from build123d import *

# Parameters (mm, degrees)
F3_DEPTH = 10
F4_R     = 5
F5_SIZE  = 15


# Not quite as in the source:
# - a fillet or chamfer that OpenCascade refuses, or shapes differently, is made with other operations: its cross-section is extruded or revolved along the edge and cut away or added


with BuildPart() as f1:
    # F0 (on Front) → F1 (revolve)
    with BuildSketch(Plane.XZ):
        Polygon((-30, 0), (0, 0), (0, 90), (-20, 90), (-20, 100), (-30, 100), (-30, 75), (-11.7123959959, 75), (-11.7123959959, 20), (-30, 20), align=None)
    revolve(axis=Axis((0, 0, 45), (0, 0, -1)))

    # F2 (on face) → F3 (cut)
    with BuildSketch(Plane.XY.offset(100)):
        with BuildLine():
            ThreePointArc((-3.2492678477, 18.4275136719), (0, 18.7117877734), (3.2492678477, 18.4275136719))
            Line((3.2492678477, 18.4275136719), (5.5579839553, 31.5208933594))
            ThreePointArc((5.5579839553, 31.5208933594), (0, 32.0071539476), (-5.5579839553, 31.5208933594))
            Line((-5.5579839553, 31.5208933594), (-3.2492678477, 18.4275136719))
        make_face()
        with BuildLine():
            ThreePointArc((-15.3277992068, 10.7326405488), (-13.2312320227, 13.2312320227), (-10.7326405488, 15.3277992068))
            Line((-10.7326405488, 15.3277992068), (-18.358549299, 26.218725588))
            ThreePointArc((-18.358549299, 26.218725588), (-22.6324756028, 22.6324756028), (-26.218725588, 18.358549299))
            Line((-26.218725588, 18.358549299), (-15.3277992068, 10.7326405488))
        make_face()
        with BuildLine():
            ThreePointArc((-18.4275136719, -3.2492678477), (-18.7117877734, 0), (-18.4275136719, 3.2492678477))
            Line((-18.4275136719, 3.2492678477), (-31.5208933594, 5.5579839553))
            ThreePointArc((-31.5208933594, 5.5579839553), (-32.0071539476, 0), (-31.5208933594, -5.5579839553))
            Line((-31.5208933594, -5.5579839553), (-18.4275136719, -3.2492678477))
        make_face()
        with BuildLine():
            ThreePointArc((-10.7326405488, -15.3277992068), (-13.2312320227, -13.2312320227), (-15.3277992068, -10.7326405488))
            Line((-15.3277992068, -10.7326405488), (-26.218725588, -18.358549299))
            ThreePointArc((-26.218725588, -18.358549299), (-22.6324756028, -22.6324756028), (-18.358549299, -26.218725588))
            Line((-18.358549299, -26.218725588), (-10.7326405488, -15.3277992068))
        make_face()
        with BuildLine():
            ThreePointArc((3.2492678477, -18.4275136719), (0, -18.7117877734), (-3.2492678477, -18.4275136719))
            Line((-3.2492678477, -18.4275136719), (-5.5579839553, -31.5208933594))
            ThreePointArc((-5.5579839553, -31.5208933594), (0, -32.0071539476), (5.5579839553, -31.5208933594))
            Line((5.5579839553, -31.5208933594), (3.2492678477, -18.4275136719))
        make_face()
        with BuildLine():
            ThreePointArc((15.3277992068, -10.7326405488), (13.2312320227, -13.2312320227), (10.7326405488, -15.3277992068))
            Line((10.7326405488, -15.3277992068), (18.358549299, -26.218725588))
            ThreePointArc((18.358549299, -26.218725588), (22.6324756028, -22.6324756028), (26.218725588, -18.358549299))
            Line((26.218725588, -18.358549299), (15.3277992068, -10.7326405488))
        make_face()
        with BuildLine():
            ThreePointArc((18.4275136719, 3.2492678477), (18.7117877734, 0), (18.4275136719, -3.2492678477))
            Line((18.4275136719, -3.2492678477), (31.5208933594, -5.5579839553))
            ThreePointArc((31.5208933594, -5.5579839553), (32.0071539476, 0), (31.5208933594, 5.5579839553))
            Line((31.5208933594, 5.5579839553), (18.4275136719, 3.2492678477))
        make_face()
        with BuildLine():
            ThreePointArc((10.7326405488, 15.3277992068), (13.2312320227, 13.2312320227), (15.3277992068, 10.7326405488))
            Line((15.3277992068, 10.7326405488), (26.218725588, 18.358549299))
            ThreePointArc((26.218725588, 18.358549299), (22.6324756028, 22.6324756028), (18.358549299, 26.218725588))
            Line((18.358549299, 26.218725588), (10.7326405488, 15.3277992068))
        make_face()
    extrude(amount=-F3_DEPTH, mode=Mode.SUBTRACT)

    # F4
    f4_edges = [f1.edges().sort_by_distance(p)[0] for p in [
        (11.712396, 0, 20),
        (30, 0, 20),
    ]]
    fillet(f4_edges, radius=F4_R)

    # F5
    f5_edges = [f1.edges().sort_by_distance(p)[0] for p in [
        (11.712396, 0, 75),
    ]]
    chamfer(f5_edges, length=F5_SIZE)

    # F6: fillet of radius 5 on 1 edges, made by hand

    # F6_s1 → F6_t2 (revolve, cut)
    with BuildSketch(Plane.XZ):
        with BuildLine():
            ThreePointArc((-26.7123959959, 75), (-29.0964606662, 76.8307454727), (-30, 79.6976270556))
            Line((-30, 79.6976270556), (-30.1, 79.6976270556))
            Line((-30.1, 79.6976270556), (-30.1, 75))
            Line((-30.1, 75), (-30, 74.9))
            ThreePointArc((-30, 74.9), (-28.3561979979, 74.9), (-26.7466439158, 74.9060474589))
            Line((-26.7466439158, 74.9060474589), (-26.7123959959, 75))
        make_face()
    revolve(axis=Axis((0, 0, 75), (0, 0, -1)), mode=Mode.SUBTRACT)


solid = f1.part
Read the model definition and answer for the solid it produces. Units are mm, in the model's axes. A direction names the side the tool comes from. Give positions to 0.01 mm unless a question says otherwise; leave off trailing zeros. Loops run counter-clockwise (first coordinate to the right, second up) from the corner with the lowest first, then second, coordinate; pieces in that order, holes last. Notation, with made-up numbers: (-4.5, -5.75) -> (48.5, -5.75) arc R20 cw to (48.5, 1.25) -> close; hole circle Ø7 at (88, 78). An arc over 180 degrees is marked (long way). Answer as CSV lines item,"result".
Item 1: Determine the mould class of faces 5 (the face through (-7.71, 18.454, 95.07)), 6 (the face through (-4.33, -24.55, 95.07)), 7 (the face through (23, -10, 100)) for opening direction Y: +Y half, -Y half, draft (parallel to the pull), parting line (faces both ways), or undercut.
Returned:
face 5,"undercut"
face 6,"-Y half"
face 7,"draft"
Item 2: Find section B-B on x = 0. Give the vertices of the cut face in (y, z), plus the area to 3 significant figures.
Returned:
outline,"(-30, 0) -> (30, 0) -> (30, 15) arc R5 ccw to (25, 20) -> (16.71, 20) arc R5 cw to (11.71, 25) -> (11.71, 60) -> (26.71, 75) arc R5 ccw to (30, 79.7) -> (30, 90) -> (-30, 90) -> (-30, 79.7) arc R5 ccw to (-26.71, 75) -> (-11.71, 60) -> (-11.71, 25) arc R5 cw to (-16.71, 20) -> (-25, 20) arc R5 ccw to (-30, 15) -> close"
area,"3,600 mm²"
Item 3: For faces 1 (the face through (5.2, -16.3, 20)), 2 (the face through (-7.6, -18.5, 95.1)), 3 (the face through (-9, -23, 100)), 4 (the face through (-24.55, 4.33, 95.07)), determine the directions among +Z, -Z, +X, -X, +Y, -Y from which every point of the face is accessible in a straight line to the end or side of a thin tool.
Returned:
face 1,"none"
face 2,"+Z"
face 3,"+Z, +X, -X, +Y, -Y"
face 4,"+Z, -X"
Item 4: Find section A-A on z = 94.5. State how many separate pieces and enclosed holes the cut face has, plus the area to 3 significant figures.
Returned:
separate pieces,"8"
enclosed holes,"0"
area,"873 mm²"
Item 5: Each of these flat-tipped pins is pushed along its axis until it touches: pin 1 (5 mm diameter, centred on x = 1, z = 75, fed in from +Y); pin 2 (6 mm diameter, centred on y = 15, z = 38, fed in from +X); pin 3 (4 mm diameter, centred on x = 15.5, z = 68, fed in from +Y). Where does it stop, or does it pass through?
Returned:
pin 1,"stops at y = 29.48"
pin 2,"passes through"
pin 3,"stops at y = 15.81"
Item 6: Consider line 1 (Z direction, x = 5.5, y = -13); line 2 (Y direction, x = -4, z = 23); line 3 (Z direction, x = 7, y = -11.5). Determine where each line is inside the solid, lowest interval first. Write a range as [from, to].
Returned:
line 1,"z = [0, 20.73], [62.4, 90]"
line 2,"y = [-11.45, 11.45]"
line 3,"z = [0, 21.2], [61.75, 90]"
